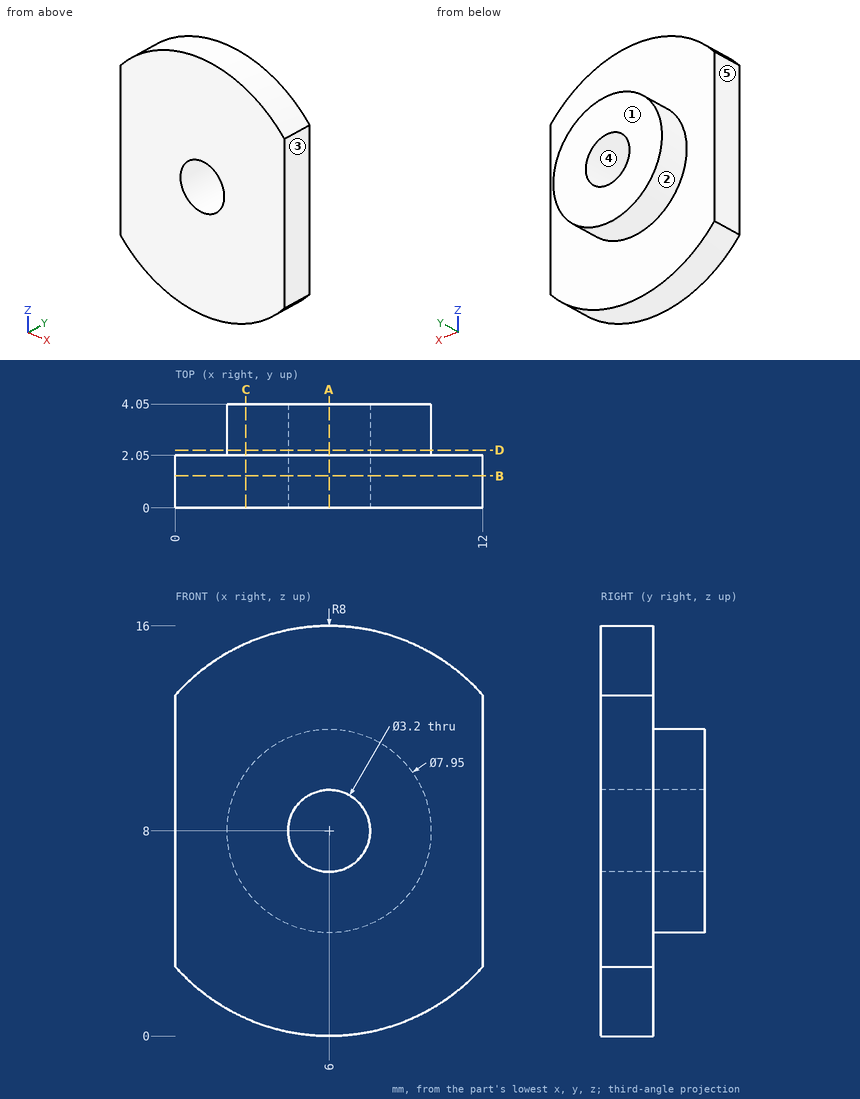
Verification items for this drawing (mm, ordinates from the low corner). A direction names the side the tool comes from. Give positions to 0.01 mm unless a question says otherwise; leave off trailing zeros. Loops run counter-clockwise (first coordinate to the right, second up) from the corner with the lowest first, then second, coordinate; pieces in that order, holes last.
(1) Section check D-D on y = 2.25. Record the cut outline in (x, z) (3 decimals).
From the geometry:
outline: circle Ø7.95 at (6, 8); hole circle Ø3.2 at (6, 8)
(2) Section check A-A on x = 6. Record the cut outline in (y, z) (3 decimals).
From the geometry:
outline: (0, 0) - (2.05, 0) - (2.05, 4.025) - (4.05, 4.025) - (4.05, 6.4) - (0, 6.4) - close; (0, 9.6) - (4.05, 9.6) - (4.05, 11.975) - (2.05, 11.975) - (2.05, 16) - (0, 16) - close
(3) Section check B-B on y = 1.25. Record the cut outline in (x, z).
From the geometry:
outline: (0, 2.71) arc R8 ccw to (12, 2.71) - (12, 13.29) arc R8 ccw to (0, 13.29) - close; hole circle Ø3.2 at (6, 8)
(4) Release check for a two-part mould opening along X. For the marked faces 3, 4 and 5 record: released by +X, released by -X, zero draft, split by the parting line, or undercut.
From the geometry:
face 3: released by +X
face 4: undercut
face 5: released by -X
(5) Thickness scan on L1, parallel to X at y = 1.55, z = 8; L2, parallel to Z at x = 6, y = 2.2 (3 decimals); L3, parallel to Y at x = 4, z = 15. Record the ranges inside material, lowest first.
From the geometry:
L1: x = 0 to 4.4, 7.6 to 12
L2: z = 4.025 to 6.4, 9.6 to 11.975
L3: y = 0 to 2.05
(6) Section check C-C on x = 2.75. Record the cut outline in (y, z).
From the geometry:
outline: (0, 0.69) - (2.05, 0.69) - (2.05, 5.71) - (4.05, 5.71) - (4.05, 10.29) - (2.05, 10.29) - (2.05, 15.31) - (0, 15.31) - close
(7) Set-up check for the marked faces 1 and 2: record each of +Z, -Z, +X, -X, +Y, -Y from which the full face is reachable in a straight line by a thin tool's end or side.
From the geometry:
face 1: +Z, -Z, +X, -X, +Y
face 2: +Y
